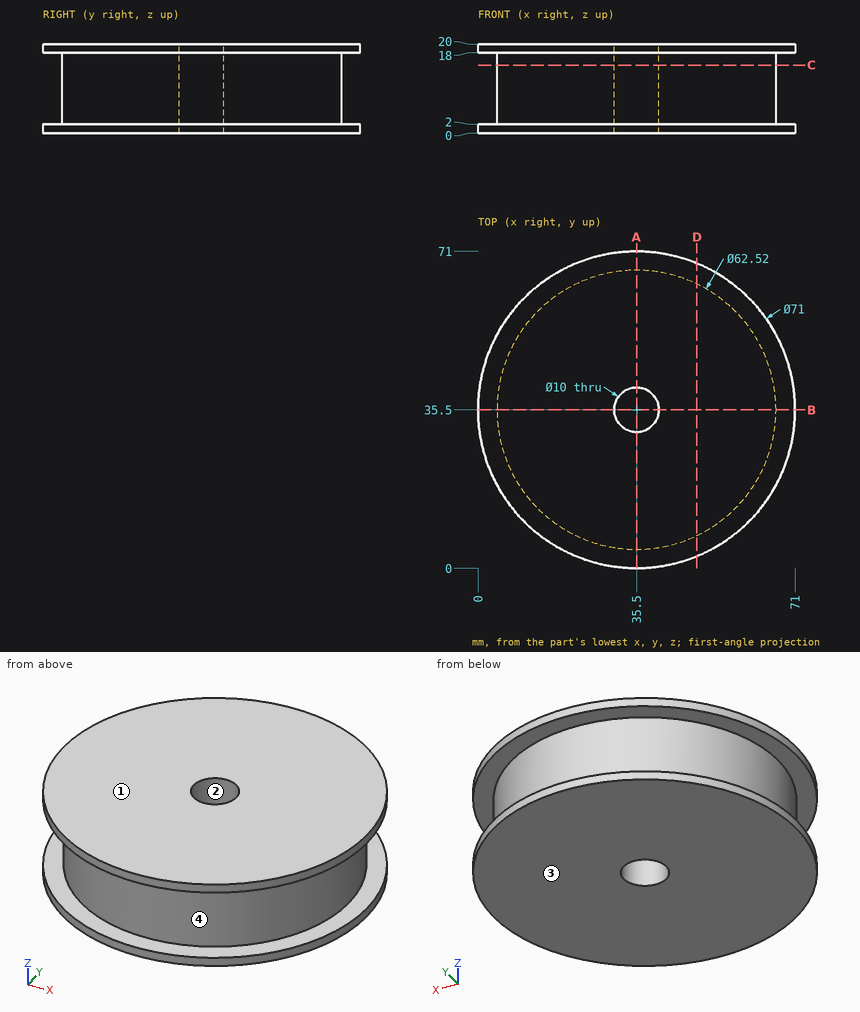
Here's the drawing with two shaded views (mm, measured from the low corner). I have some questions. Give positions to 0.01 mm unless a question says otherwise; leave off trailing zeros. Loops run counter-clockwise (first coordinate to the right, second up) from the corner with the lowest first, then second, coordinate; pieces in that order, holes last. Notation, with made-up numbers: (37.5, -12) -> (77.5, -12) arc R32 ccw to (77.5, 22) -> close; hole circle Ø4 at (88.25, 10.5). An arc over 180 degrees is marked (long way). Use one line per item in the form item = value.
1) Will these pins go through, and if not, where does the flat tip stop? pin 1 (10 mm diameter, centred on x = 54.5, z = 9, fed in from -Y); pin 2 (2 mm diameter, centred on y = 56, z = 4.5, fed in from +X); pin 3 (8 mm diameter, centred on x = 33, z = 17, fed in from +Y).
Answers:
pin_1 = 7.55
pin_2 = 59.93
pin_3 = 71
2) If we section it at D-D (x = 49): Please give me the cut outline in (y, z).
Answers:
outline = (2.67, 0) -> (68.33, 0) -> (68.33, 2) -> (63.69, 2) -> (63.69, 18) -> (68.33, 18) -> (68.33, 20) -> (2.67, 20) -> (2.67, 18) -> (7.31, 18) -> (7.31, 2) -> (2.67, 2) -> close
3) I need wall thicknesses on line 1 along Y through (x, z) = (35.5, 12.5); line 2 along Y through (x, z) = (34, 5); line 3 along Z through (x, y) = (67, 25). Which ranges of each line are inside material? Lowest first, please.
Answers:
line_1 = 4.24 to 30.5, 40.5 to 66.76
line_2 = 4.28 to 30.73, 40.27 to 66.72
line_3 = 0 to 2, 18 to 20
4) We'd pull the mould along Z, two halves only. Please class the marked faces 1, 2, 3 and 4: released by +Z, released by -Z, zero draft, split by the parting line, or undercut.
Answers:
face_1 = released by +Z
face_2 = zero draft
face_3 = released by -Z
face_4 = undercut
5) If we section it at A-A (x = 35.5): Please give me the cut outline in (y, z), plus the area to 3 significant figures.
Answers:
outline = (0, 0) -> (30.5, 0) -> (30.5, 20) -> (0, 20) -> (0, 18) -> (4.24, 18) -> (4.24, 2) -> (0, 2) -> close; (40.5, 0) -> (71, 0) -> (71, 2) -> (66.76, 2) -> (66.76, 18) -> (71, 18) -> (71, 20) -> (40.5, 20) -> close
area = 1,080 mm²
6) If we section it at C-C (z = 15.25): Please give me the cut outline in (x, y), plus the area to 3 significant figures.
Answers:
outline = circle Ø62.52 at (35.5, 35.5); hole circle Ø10 at (35.5, 35.5)
area = 2,990 mm²
